Geometry: final body of the model. Coordinates: model frame, mm. Face numbers are marked on the shaded views. Give positions to 0.01 mm unless a question says otherwise; leave off trailing zeros. Loops run counter-clockwise (first coordinate to the right, second up) from the corner with the lowest first, then second, coordinate; pieces in that order, holes last.
1. Draft query along X for the marked faces 1, 2, 3 and 4. Return one class per face: +X half, -X half, draft (parallel to the pull), parting line (faces both ways), or undercut.
2. Section A-A, the plane z = 2.15. Output: boundary loops of the cut face in (x, y).
3. Section B-B, the plane z = 0.2. Output: boundary loops of the cut face in (x, y).
4. Material intervals for line 1 along X through (y, z) = (0.5, 2.5); line 2 along X through (y, z) = (-1, 1.9); line 3 along Y through (x, z) = (-1, 0.8), sorted ascending.
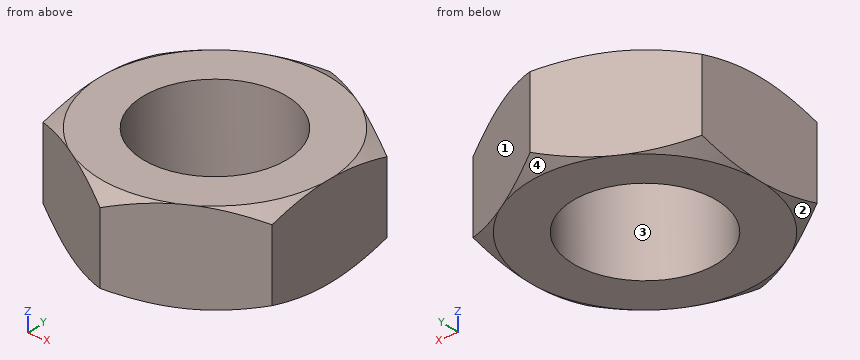
from build123d import *

# Parameters (mm, degrees)
EXTRUDE1_DEPTH     = 3.2
SKETCH2_R          = 2.5
CUT_EXTRUDE1_DEPTH = 4.2


with BuildPart() as part:
    # Sketch1 → Extrude1 (new body)
    with BuildSketch(Plane.XY):
        Polygon((0, 4.618802154), (-4, 2.309401077), (-4, -2.309401077), (0, -4.618802154), (4, -2.309401077), (4, 2.309401077), align=None)
    extrude(amount=EXTRUDE1_DEPTH)

    # Sketch2 → Cut-Extrude1 (cut, through all)
    with BuildSketch(Plane.XY.offset(3.2)):
        Circle(SKETCH2_R)
    extrude(amount=-CUT_EXTRUDE1_DEPTH, mode=Mode.SUBTRACT)

    # Sketch3 → Cut-Revolve1 (revolve, cut)
    with BuildSketch(Plane(origin=(0, 0, 0), x_dir=(0, 0, -1), z_dir=(1, 0, 0))):
        Polygon((-3.2, 5.618802154), (-2.265384141, 5.618802154), (-3.2, 4), align=None)
    cut_revolve1 = revolve(axis=Axis((0, 0, 0), (0, 0, 1)), mode=Mode.SUBTRACT)

    # Mirror1: Cut-Revolve1 across plane
    add(cut_revolve1.mirror(Plane.XY.offset(1.6)), mode=Mode.SUBTRACT)


solid = part.part
Answers below:
1. face 1: +X half
1. face 2: -X half
1. face 3: undercut
1. face 4: parting line
2. outline: (-4, -2.31) - (0, -4.62) - (4, -2.31) - (4, 2.31) - (0, 4.62) - (-4, 2.31) - close; hole circle Ø5 at (0, 0)
3. outline: (-4, -1.7) arc R4.35 ccw to (-3.47, -2.61) - (-0.53, -4.31) arc R4.35 ccw to (0.53, -4.31) - (3.47, -2.61) arc R4.35 ccw to (4, -1.7) - (4, 1.7) arc R4.35 ccw to (3.47, 2.61) - (0.53, 4.31) arc R4.35 ccw to (-0.53, 4.31) - (-3.47, 2.61) arc R4.35 ccw to (-4, 1.7) - close; hole circle Ø5 at (0, 0)
4. line 1: x = -4 to -2.45, 2.45 to 4
4. line 2: x = -4 to -2.29, 2.29 to 4
4. line 3: y = -4.04 to -2.29, 2.29 to 4.04
